Here's how the part is built. I have some questions about the finished solid (model axes, mm). Coordinates: 2 decimals unless noted, no trailing zeros. Write each loop counter-clockwise with the first axis right and the second up, starting at its lowest first coordinate (ties: lowest second). Pieces come first, ordered by that corner, then holes.
Item 1: Please list where these lines run through material, in increasing order: line 1 (X direction, y = -5.5, z = 0.9); line 2 (Y direction, x = -8, z = 0.55); line 3 (Y direction, x = 7.5, z = 0.7).
Item 2: If we mould it in two halves opening along X, with no side actions, what happens to faces 1 (the face through (0, 9.5, 1)), 2 (the face through (-6.56, 5.73, 0.74)), 3 (the face through (-12.5, 0, 1)), 4 (the face through (7.29, -4.726, 0.74))? For each: pulls with the +X half, pulls with the -X half, needs draft (parallel to the pull), parting line crosses it, or undercut.
Item 3: I want a section at A-A (z = 0.45). Please give me the cut outline in (x, y), and give its area (3 significant figures).
Item 4: I want a section at C-C (x = 8). Please give me the cut outline in (y, z), and give its area (3 significant figures).
Item 5: I want a section at B-B (y = -5.5). Please give me the cut outline in (x, z), and give its area (3 significant figures).
Autodesk Inventor part; units mm, degrees
ref_plane "YZ Plane" through (0, 0, 0) normal (1, 0, 0) x (0, 1, 0)
ref_plane "XZ Plane" through (0, 0, 0) normal (0, 1, 0) x (-1, 0, 0)
ref_plane "XY Plane" through (0, 0, 0) normal (0, 0, 1) x (1, 0, 0)
sketch "スケッチ1" plane through (0, 0, 0) normal (0, 0, 1) x (1, 0, 0)
  line L0 (-12.5, 9.5) -> (12.5, 9.5)
  line L1 (12.5, 9.5) -> (12.5, -9.5)
  line L2 (12.5, -9.5) -> (-12.5, -9.5)
  line L3 (-12.5, -9.5) -> (-12.5, 9.5)
  line L4 (-12.5, 9.5) -> (12.5, -9.5) construction
  line L5 (12.5, 9.5) -> (-12.5, -9.5) construction
  point P0 (0, 0)
  dimension "d0" = 25
  dimension "d1" = 19
extrude "押し出し1" add sketch "スケッチ1" along normal blind 1.5
sketch "スケッチ2" plane through (0, 0, 1.5) normal (0, 0, 1) x (1, 0, 0)
  line L0 (-12.5, -9.5) -> (12.5, -9.5)
  line L1 (-12.5, 9.5) -> (-12.5, -9.5)
  line L2 (12.5, -9.5) -> (12.5, 9.5)
  point P0 (0, 0)
  point P1 (-8, -5.5)
  point P2 (8, -5.5)
  dimension "d4" = 4
  dimension "d5" = 4.5
  dimension "d6" = 4.5
  dimension "d7" = 4
hole "穴1" at (-8, -5.5, 1.5) at (8, -5.5, 1.5) direction (0, 0, -1) diameter 2.1 end through all
sketch "スケッチ3" plane through (0, 0, 1.5) normal (0, 0, 1) x (1, 0, 0)
  line L0 (12.5, -9.5) -> (12.5, 9.5)
  line L1 (12.5, 9.5) -> (-12.5, 9.5)
  line L2 (-12.5, 9.5) -> (-12.5, -9.5)
  point P0 (0, 0)
  point P1 (-7.5, 4.5)
  point P2 (7.5, 4.5)
  dimension "d15" = 5
  dimension "d16" = 5
  dimension "d17" = 5
  dimension "d18" = 5
hole "穴2" at (-7.5, 4.5, 1.5) at (7.5, 4.5, 1.5) direction (0, 0, -1) diameter 3.1 end through all
properties part number "servo catch back c"
Answer:
1. line 1: x = -12.5 to -9.05, -6.95 to 6.95, 9.05 to 12.5
1. line 2: y = -9.5 to -6.55, -4.45 to 3.03, 5.97 to 9.5
1. line 3: y = -9.5 to -6.42, -4.58 to 2.95, 6.05 to 9.5
2. face 1: needs draft
2. face 2: undercut
2. face 3: pulls with the -X half
2. face 4: undercut
3. outline: (-12.5, -9.5) - (12.5, -9.5) - (12.5, 9.5) - (-12.5, 9.5) - close; hole circle Ø2.1 at (-8, -5.5); hole circle Ø3.1 at (-7.5, 4.5); hole circle Ø3.1 at (7.5, 4.5); hole circle Ø2.1 at (8, -5.5)
3. area: 453 mm2
4. outline: (-9.5, 0) - (-6.55, 0) - (-6.55, 1.5) - (-9.5, 1.5) - close; (-4.45, 0) - (3.03, 0) - (3.03, 1.5) - (-4.45, 1.5) - close; (5.97, 0) - (9.5, 0) - (9.5, 1.5) - (5.97, 1.5) - close
4. area: 20.9 mm2
5. outline: (-12.5, 0) - (-9.05, 0) - (-9.05, 1.5) - (-12.5, 1.5) - close; (-6.95, 0) - (6.95, 0) - (6.95, 1.5) - (-6.95, 1.5) - close; (9.05, 0) - (12.5, 0) - (12.5, 1.5) - (9.05, 1.5) - close
5. area: 31.2 mm2
